```python
from build123d import *

# Parameters (mm, degrees)
SKETCH1_R           = 2.159
SKETCH1_R_2         = 11.112499999999992
SKETCH1_R_3         = 2.032000000000007
SKETCH1_R_4         = 2.0320000000000227
SKETCH1_R_5         = 2.159000000000001
BOSS_EXTRUDE1_DEPTH = 6.35
SKETCH2_R           = 12.573000000000004
CUT_EXTRUDE1_DEPTH  = 1.5875
BOSS_EXTRUDE2_DEPTH = 31.75
FILLET1_R           = 3.175


with BuildPart() as part:
    # Sketch1 → Boss-Extrude1 (new body)
    with BuildSketch(Plane(origin=(0, 0, 0), x_dir=(0, 0, -1), z_dir=(1, 0, 0))):
        with BuildLine():
            Line((1.7528307479226393, 4.428203994751931), (-74.44716925207737, 34.59070399475192))
            ThreePointArc((-74.44716925207737, 34.59070399475192), (-76.54899129091997, 34.912195919620736), (-78.58125, 34.28694598552338))
            Line((-78.58125, 34.28694598552338), (-104.70274124164806, 19.205695985523498))
            ThreePointArc((-104.70274124164806, 19.205695985523498), (-106.99949191381467, 15.974399461853373), (-106.05477455872966, 12.124224142081344))
            Line((-106.05477455872966, 12.124224142081344), (-88.64427772360533, -9.856752859729227))
            ThreePointArc((-88.64427772360533, -9.856752859729227), (-82.04819337667968, -14.758531743671528), (-73.88489583333335, -15.705283114209777))
            Line((-73.88489583333335, -15.705283114209777), (0.6945312500000005, -4.711584934262932))
            ThreePointArc((0.6945312500000005, -4.711584934262932), (4.730891100411702, -0.5477916082283132), (1.7528307479226393, 4.428203994751931))
        make_face()
        Circle(SKETCH1_R, mode=Mode.SUBTRACT)
        with Locations((-76.2, -9.33e-15)):
            Circle(SKETCH1_R_2, mode=Mode.SUBTRACT)
        with Locations((-76.2, 30.162499999999987)):
            Circle(SKETCH1_R_3, mode=Mode.SUBTRACT)
        with Locations((-102.32149124164806, 15.081250000000113)):
            Circle(SKETCH1_R_4, mode=Mode.SUBTRACT)
        with Locations((-17.960512242138307, -2.2e-15)):
            Circle(SKETCH1_R_5, mode=Mode.SUBTRACT)
    extrude(amount=BOSS_EXTRUDE1_DEPTH)

    # Sketch2 → Cut-Extrude1 (cut)
    with BuildSketch(Plane(origin=(6.35, 0, 0), x_dir=(0, 0, -1), z_dir=(1, 0, 0))):
        with Locations((-76.2, -9.33e-15)):
            Circle(SKETCH2_R)
    extrude(amount=-CUT_EXTRUDE1_DEPTH, mode=Mode.SUBTRACT)

    # Sketch3 → Boss-Extrude2 (add)
    with BuildSketch(Plane(origin=(6.35, 0, 0), x_dir=(0, 0, -1), z_dir=(1, 0, 0))):
        with BuildLine():
            Line((-78.58125000000001, 34.286945985523374), (-104.70274124164803, 19.20569598552344))
            ThreePointArc((-104.70274124164803, 19.20569598552344), (-106.9994919138146, 15.974399461853357), (-106.05477455872966, 12.124224142081344))
            Line((-106.05477455872966, 12.124224142081344), (-101.58067912721546, 6.475620904888487))
            ThreePointArc((-101.58067912721546, 6.475620904888487), (-90.28737650298505, 22.08298807511437), (-71.374, 25.745334782490193))
            Line((-71.374, 25.745334782490193), (-71.374, 33.37424116580463))
            Line((-71.374, 33.37424116580463), (-71.46391508012837, 30.663405062626204))
            ThreePointArc((-71.46391508012837, 30.663405062626204), (-74.0392538140866, 34.40662325104498), (-78.58125000000001, 34.286945985523374))
        make_face()
        Polygon((-76.19999999999999, 33.901997693541205), (-79.4385, 32.03224884677059), (-79.4385, 28.292751153229368), (-76.20000000000002, 26.42300230645877), (-72.9615, 28.292751153229386), (-72.9615, 32.03224884677061), align=None, mode=Mode.SUBTRACT)
        Polygon((-102.32149124164808, 18.820747693541325), (-105.55999124164805, 16.950998846770727), (-105.55999124164805, 13.211501153229527), (-102.32149124164805, 11.341752306458922), (-99.08299124164807, 13.211501153229516), (-99.08299124164807, 16.95099884677072), align=None, mode=Mode.SUBTRACT)
    extrude(amount=BOSS_EXTRUDE2_DEPTH)

    # Fillet1
    fillet1_edges = [part.edges().sort_by_distance(p)[0] for p in [
        (22.225, 25.745334782490197, 71.374),
        (22.225, 6.475620904888487, 101.58067912721546),
    ]]
    fillet(fillet1_edges, radius=FILLET1_R)


with BuildPart() as body_2:
    # Mirror1: mirrored copy
    add(part.part.mirror(Plane(origin=(6.35, 0, 0), x_dir=(0, 0, 1), z_dir=(1, 0, 0))))


solid = body_2.part
```
Input: part model. Units: mm. Frame: model coordinates. A direction names the side the tool comes from. Coordinates: 2 decimals unless noted, no trailing zeros. Loops run counter-clockwise (first coordinate to the right, second up) from the corner with the lowest first, then second, coordinate; pieces in that order, holes last.
Q1. Line query: line 1 along Y through (x, z) = (7.1, 76.2) (1 decimal); line 2 along Y through (x, z) = (8, 76); line 3 along X through (y, z) = (8.5, 96). Output: solid intervals per line, ascending.
Results are:
line 1: y = -15.9 to -12.6, 12.6 to 28.1, 32.2 to 34.9
line 2: y = -15.87 to -11.11, 11.11 to 28.14, 32.18 to 34.92
line 3: x = 6.35 to 12.7
Q2. Section C-C, the plane x = -23. Give the number of separate pieces and of enclosed holes in the cut face, and give its area (3 significant figures).
Results are:
separate pieces: 1
enclosed holes: 2
area: 190 mm2
Q3. Section D-D, the plane y = 0. Return the cut outline in (x, z), and give its area (3 significant figures).
Results are:
outline: (6.35, -4.76) - (12.7, -4.76) - (12.7, -2.16) - (6.35, -2.16) - close; (6.35, 2.16) - (12.7, 2.16) - (12.7, 15.8) - (6.35, 15.8) - close; (6.35, 20.12) - (12.7, 20.12) - (12.7, 65.09) - (7.94, 65.09) - (7.94, 63.63) - (6.35, 63.63) - close; (6.35, 88.77) - (7.94, 88.77) - (7.94, 87.31) - (12.7, 87.31) - (12.7, 96.45) - (6.35, 96.45) - close
area: 442 mm2
Q4. Set-up query: faces 1 (the flat face through (-9.3, 27.37, 77.84)), 2 (the cylindrical face through (10.4, 0.5, 87.3)). Return all of +Z, -Z, +X, -X, +Y, -Y with unobstructed straight access to the full face (end or side cutting, diameter ignored); none if empty.
Results are:
face 1: -X
face 2: +X, -X
Q5. Section B-B, the plane z = 67. Return the cut outline in (x, y).
Results are:
outline: (6.35, -14.69) - (12.7, -14.69) - (12.7, -6.23) - (7.94, -6.23) - (7.94, -8.57) - (6.35, -8.57) - close; (6.35, 8.57) - (7.94, 8.57) - (7.94, 6.23) - (12.7, 6.23) - (12.7, 31.64) - (6.35, 31.64) - close
Q6. Contact query for flat-ended pins moving along their axis: pin 1 (4 mm diameter, centred on x = -12.5, y = 15, fed in from -Z); pin 2 (7 mm diameter, centred on y = 0, z = 0, fed in from -X); pin 3 (5 mm diameter, centred on y = 2, z = 82.5, fed in from -X); pin 4 (1.5 mm diameter, centred on x = -14.5, z = 86.5, fed in from -Y). Output: stop coordinate, or through.
Results are:
pin 1: stops at z = 96.13
pin 2: stops at x = 6.35
pin 3: passes through
pin 4: stops at y = 23.75
Q7. Mould query, pull axis Z, two halves, no side actions, for faces 3 (the cylindrical face through (-6.08, 16.03, 106.99)), 4 (the flat face through (-9, 30, 71.374)), 5 (the flat face through (6.35, 33, 72)), 6 (the cylindrical face through (9.569, 15.692, 100.383)). Classes: +Z half, -Z half, draft (parallel to the pull), parting line (faces both ways), or undercut.
Results are:
face 3: +Z half
face 4: -Z half
face 5: undercut
face 6: undercut
Q8. Section A-A, the plane y = -8. Return the cut outline in (x, z).
Results are:
outline: (6.35, 21.61) - (12.7, 21.61) - (12.7, 68.49) - (7.94, 68.49) - (7.94, 66.5) - (6.35, 66.5) - close; (6.35, 85.9) - (7.94, 85.9) - (7.94, 83.91) - (12.7, 83.91) - (12.7, 90.11) - (6.35, 90.11) - close
